Build history of the part. All positions in model axes, mm. Face numbers are marked on the shaded views. A direction names the side the tool comes from. Give positions to 0.01 mm unless a question says otherwise; leave off trailing zeros. Loops run counter-clockwise (first coordinate to the right, second up) from the corner with the lowest first, then second, coordinate; pieces in that order, holes last. Notation, with made-up numbers: (20.25, -12.5) -> (54.25, -12.5) arc R26 cw to (54.25, 15.5) -> close; hole circle Ø4 at (83, -17.5). An arc over 180 degrees is marked (long way). One line per question, with ' | ' between items. Start each with the question number.
(1) Slice it at A-A, the plane y = 0. Write the cut outline in (x, z).
(2) 3-axis set-ups, long thin cutter, end or side, ignore diameter. For the marked faces 4, 5 and 6: which of +Z, -Z, +X, -X, +Y, -Y reach the whole face in a straight line?
(3) Flat gauge pin, fed straight in: pin 1 Ø0.5 at (x, y) = (0, 0.5) entering from +Z. Where does the tip first touch, or does it go through?
(4) Mould opens along Y. For the marked faces 1, 2 and 3 say: pulls with the +Y half, pulls with the -Y half, needs draft (parallel to the pull), parting line crosses it, or undercut.
(5) Slice it at B-B, the plane z = -2.5. Write the cut outline in (x, y), then the cut area to 3 significant figures.
(6) Drill centre lines: L1, parallel to Z at x = -0.4, y = -0.05; L2, parallel to Y at x = -0.45, z = -3; L3, parallel to Z at x = 1.7, y = -0.9. Where is each one in solid material? Low to high. Write a range as from..to.
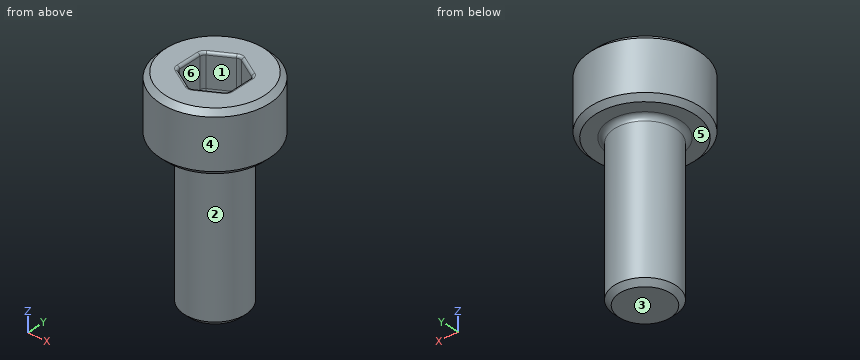
```python
from build123d import *

# Parameters (mm, degrees)
SCHNITT_LINEAR_AUSTRAGEN1_DEPTH = 1.5
FASE1_SIZE                      = 0.2
VERRUNDUNG1_R                   = 0.2
VERRUNDUNG2_R                   = 0.1


with BuildPart() as part:
    # Skizze1 → Rotation1 (revolve)
    with BuildSketch(Plane(origin=(0, 0, 0), x_dir=(0, 0, -1), z_dir=(1, 0, 0))):
        Polygon((-2.35, 0), (-2.35, 2.15), (0, 2.15), (0, 1.21), (6, 1.21), (6, 0), align=None)
    revolve(axis=Axis((0, 0, 21.919879518), (0, 0, -1)))

    # Skizze2 → Schnitt-Linear austragen1 (cut)
    with BuildSketch(Plane.XY.offset(2.35)):
        Polygon((1, -0.577350269), (1, 0.577350269), (0, 1.154700538), (-1, 0.577350269), (-1, -0.577350269), (0, -1.154700538), align=None)
    extrude(amount=-SCHNITT_LINEAR_AUSTRAGEN1_DEPTH, mode=Mode.SUBTRACT)

    # Fase1
    fase1_edges = [part.edges().sort_by_distance(p)[0] for p in [
        (0, -1.21, -6),
        (0, -2.15, 0),
        (0, -2.15, 2.35),
    ]]
    chamfer(fase1_edges, length=FASE1_SIZE)

    # Verrundung1
    verrundung1_edges = [part.edges().sort_by_distance(p)[0] for p in [
        (0.5, -0.866025404, 0.85),
        (1, -0.577350269, 1.6),
        (-0.5, -0.866025404, 0.85),
        (0, -1.154700538, 1.6),
        (-1, 0, 0.85),
        (-1, -0.577350269, 1.6),
        (-0.5, 0.866025404, 0.85),
        (-1, 0.577350269, 1.6),
        (0.5, 0.866025404, 0.85),
        (0, 1.154700538, 1.6),
        (1, 0, 0.85),
        (1, 0.577350269, 1.6),
        (0, -1.21, 0),
    ]]
    fillet(verrundung1_edges, radius=VERRUNDUNG1_R)

    # Verrundung2
    verrundung2_edges = [part.edges().sort_by_distance(p)[0] for p in [
        (-0.5, -0.866025404, 2.35),
        (-1, 0, 2.35),
        (-0.5, 0.866025404, 2.35),
        (0.5, 0.866025404, 2.35),
        (1, 0, 2.35),
        (0.5, -0.866025404, 2.35),
        (-0.973205081, -0.561880215, 2.35),
        (0, -1.123760431, 2.35),
        (0.973205081, -0.561880215, 2.35),
        (0.973205081, 0.561880215, 2.35),
        (0, 1.123760431, 2.35),
        (-0.973205081, 0.561880215, 2.35),
    ]]
    fillet(verrundung2_edges, radius=VERRUNDUNG2_R)


solid = part.part
```
Final values:
1) outline: (-2.15, 0.2) -> (-1.95, 0) -> (-1.41, 0) arc R0.2 cw to (-1.21, -0.2) -> (-1.21, -5.8) -> (-1.01, -6) -> (1.01, -6) -> (1.21, -5.8) -> (1.21, -0.2) arc R0.2 cw to (1.41, 0) -> (1.95, 0) -> (2.15, 0.2) -> (2.15, 2.15) -> (1.95, 2.35) -> (1.1, 2.35) arc R0.1 ccw to (1, 2.25) -> (1, 1.05) arc R0.2 cw to (0.8, 0.85) -> (-0.8, 0.85) arc R0.2 cw to (-1, 1.05) -> (-1, 2.25) arc R0.1 ccw to (-1.1, 2.35) -> (-1.95, 2.35) -> (-2.15, 2.15) -> close
2) face 4: +Z, -Z | face 5: -Z | face 6: +Z
3) pin 1: z = 0.85
4) face 1: undercut | face 2: parting line crosses it | face 3: needs draft
5) outline: circle Ø2.42 at (0, 0) | area: 4.60 mm2
6) L1: -6..0.85 | L2: -1.12..1.12 | L3: 0..2.35
